Print and shaded views of the part. All mm, measured from the part's lowest x, y and z. Round coordinates to 2 decimals unless told otherwise and drop trailing zeros. Loops run counter-clockwise (first coordinate to the right, second up) from the corner with the lowest first, then second, coordinate; pieces in that order, holes last. Notation, with made-up numbers: (-7.5, 31) - (2.5, 31) arc R14 cw to (2.5, 56) - close; hole circle Ø10 at (88.5, 65.25). An arc over 180 degrees is marked (long way). Use one line per item in the form item = value.
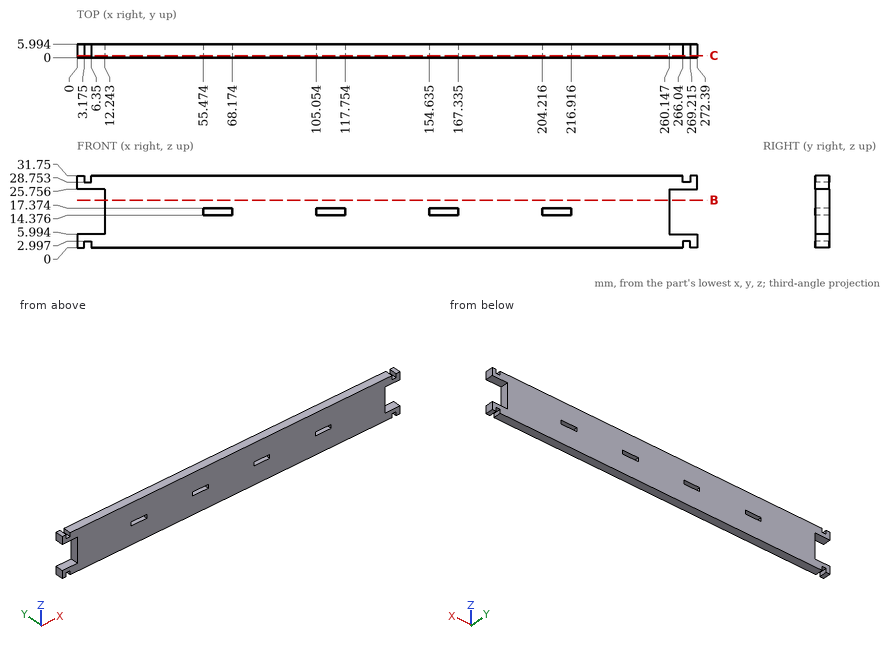
1) Slice it at B-B (z = 21). Write the cut outline in (x, y) (1 decimal), plus the area to 3 significant figures.
Report:
outline = (12.2, 0) - (260.1, 0) - (260.1, 6) - (12.2, 6) - close
area = 1,490 mm^2
2) Slice it at C-C (y = 0.9). State how many separate pieces and enclosed holes the cut face has, plus the area to 3 significant figures.
Report:
separate_pieces = 1
enclosed_holes = 4
area = 7,970 mm^2
3) Drill centre lines: probe 1 along Z at (x, y) = (165, 4.5); probe 2 along X at (y, z) = (0.65, 19). Where is each one in solid material? Low to high.
Report:
probe_1 = 0 to 14.38, 17.37 to 31.75
probe_2 = 12.24 to 260.15
4) Flat gauge pins, fed straight in: pin 1 (1 mm diameter, centred on x = 4, y = 3.5, fed in from +Z); pin 2 (1.5 mm diameter, centred on x = 213.5, z = 25, fed in from -Y); pin 3 (1.8 mm diameter, centred on y = 3, z = 18.5, fed in from -X); pin 4 (0.9 mm diameter, centred on y = 2.5, z = 16.5, fed in from +X). Where does each tip first touch, or does it go through?
Report:
pin_1 = 28.75
pin_2 = 0
pin_3 = 12.24
pin_4 = 260.15
